from build123d import *

# Parameters (mm, degrees)
SKETCH1_W             = 40
SKETCH1_H             = 30
BOSS_EXTRUDE1_DEPTH   = 6.35
CUT_EXTRUDE1_DEPTH    = 7.35
F_6_CLEARANCE_HOLE1_D = 3.6576


with BuildPart() as part:
    # Sketch1 → Boss-Extrude1 (new body)
    with BuildSketch(Plane(origin=(0, 0, 0), x_dir=(1, 0, 0), z_dir=(0, 1, 0))):
        Rectangle(SKETCH1_W, SKETCH1_H)
    extrude(amount=BOSS_EXTRUDE1_DEPTH)

    # Sketch2 → Cut-Extrude1 (cut, through all)
    with BuildSketch(Plane(origin=(0, 6.35, 0), x_dir=(1, 0, 0), z_dir=(0, 1, 0))):
        Polygon((-12.7, 15), (-12.5, 4.97), (12.5, 4.97), (12.7, 15), align=None)
    extrude(amount=-CUT_EXTRUDE1_DEPTH, mode=Mode.SUBTRACT)

    # #6 Clearance Hole1 (through all)
    with Locations(Plane(origin=(0, 6.35, 5.4948), x_dir=(0, 0, 1), z_dir=(0, 1, 0))):
        with Locations((0, 0)):
            Hole(F_6_CLEARANCE_HOLE1_D / 2)


solid = part.part
Build history of the part. All positions in model axes, mm. A direction names the side the tool comes from. Coordinates: 2 decimals unless noted, no trailing zeros. Order: outer loops, then holes, each group sorted by start corner. A loop starts at its lowest first (then second) coordinate and runs counter-clockwise, first axis right, second up. Notation, with made-up numbers: (-15, 37.25) - (-2, 37.25) arc R9 cw to (-2, 53.25) - close; hole circle Ø9 at (44.25, -39.75). An arc over 180 degrees is marked (long way). Write each question's results on one line, items separated by ' | '. Start each with the question number.
Item 1: Mould opens along X. For faces 3 (the face through (-0.7, 3.131, 3.805)), 4 (the face through (20, 3, 0)), 5 (the face through (16, 3, -15)) say: released by +X, released by -X, zero draft, split by the parting line, or undercut.
Item 2: Band-saw the part on C-C on z = 5.75. Write the cut outline in (x, y).
Item 3: Band-saw the part on D-D on x = 10. Write the cut outline in (y, z), and give its area (3 significant figures).
Item 4: Band-saw the part on B-B on y = 1.5. Write the cut outline in (x, z).
Item 5: Tool access for faces 1 (the face through (-16, 3, -15)), 2 (the face through (0, 3, -4.97)): list every direction of +Z, -Z, +X, -X, +Y, -Y with a clear straight run to the whole face (end or side of a thin tool).
Item 6: Flat gauge pin, fed straight in: pin 1 (1.5 mm diameter, centred on x = 1, z = 4.5, fed in from +Y). Where does the tip first touch, or does it go through?
Item 7: Wall check: probe 1 along Z at (x, y) = (10.5, 4.5); probe 2 along X at (y, z) = (5.25, -13.5); probe 3 along X at (y, z) = (3.5, -5.75). Give the ranges that are in metal, low to high. Write a range as [from, to].
Item 8: Band-saw the part on A-A on x = 0. Write the cut outline in (y, z).
Numbers:
1) face 3: undercut | face 4: released by +X | face 5: zero draft
2) outline: (-20, 0) - (-1.81, 0) - (-1.81, 6.35) - (-20, 6.35) - close; (1.81, 0) - (20, 0) - (20, 6.35) - (1.81, 6.35) - close
3) outline: (0, -4.97) - (6.35, -4.97) - (6.35, 15) - (0, 15) - close | area: 127 mm^2
4) outline: (-20, -15) - (-12.7, -15) - (-12.5, -4.97) - (12.5, -4.97) - (12.7, -15) - (20, -15) - (20, 15) - (-20, 15) - close; hole circle Ø3.66 at (0, 5.49)
5) face 1: -Z, +X, -X, +Y, -Y | face 2: -Z, +Y, -Y
6) pin 1: y = 6.35
7) probe 1: [-4.97, 15] | probe 2: [-20, -12.67], [12.67, 20] | probe 3: [-20, -12.52], [12.52, 20]
8) outline: (0, -4.97) - (6.35, -4.97) - (6.35, 3.67) - (0, 3.67) - close; (0, 7.32) - (6.35, 7.32) - (6.35, 15) - (0, 15) - close
